Geometry: see drawing. Coordinates: mm, zero at the bounding-box minimum. A direction names the side the tool comes from. Give positions to 0.01 mm unless a question says otherwise; leave off trailing zeros. Loops run counter-clockwise (first coordinate to the right, second up) from the corner with the lowest first, then second, coordinate; pieces in that order, holes last. Notation, with made-up numbers: (65.25, 36.25) - (108.25, 36.25) arc R36 ccw to (108.25, 72.25) - close; hole circle Ø4 at (-11.75, 47.5). An arc over 180 degrees is marked (long way). One line per question, with ' | ' between items. Start each with the question number.
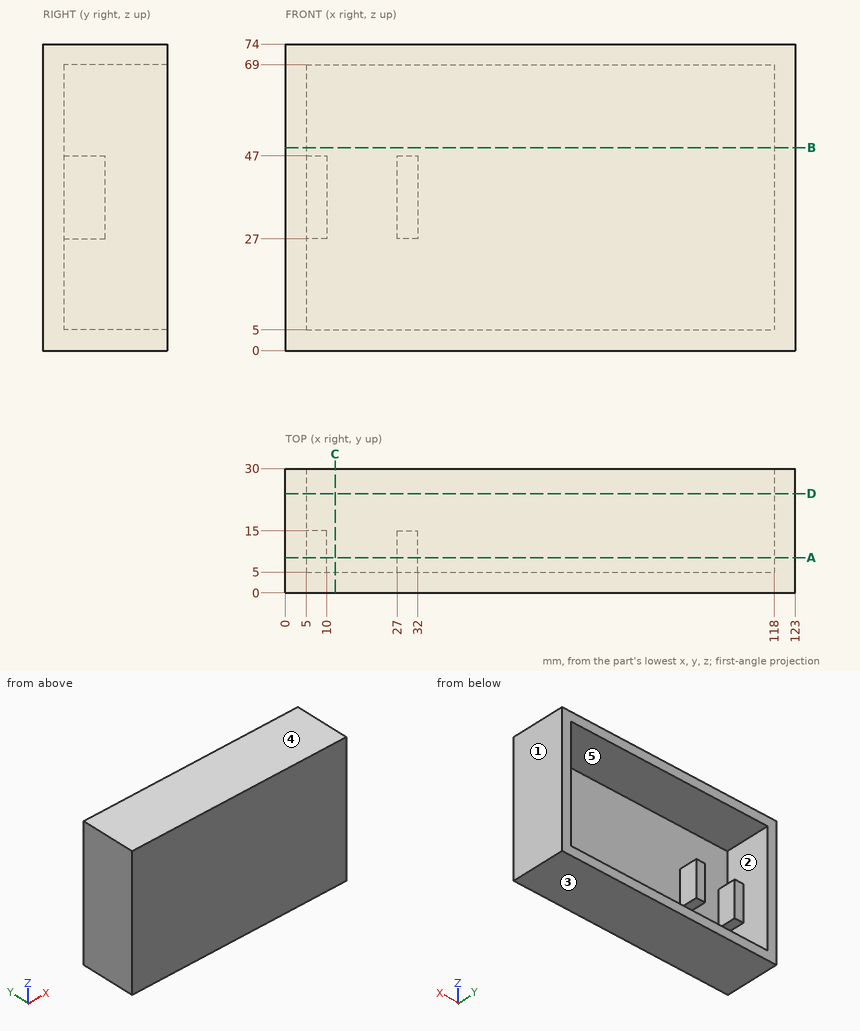
Q1. First-contact query: pin 1 (2.5 mm diameter, centred on x = 29, y = 11, fed in from -Z); pin 2 (6 mm diameter, centred on x = 68.5, z = 46.5, fed in from +Y); pin 3 (1.5 mm diameter, centred on x = 7.5, z = 37, fed in from +Y). Flat tips, straight axial feed; report the tip coordinate or a pass-through.
Q2. Section C-C, the plane x = 12. Output: boundary loops of the cut face in (y, z).
Q3. Access query for the marked faces 4 and 5. Directions: +Z, -Z, +X, -X, +Y, -Y. A direction counts if a zero-diameter tool reaches every point of the face in a straight line with its end or side. Return the directions, or none.
Q4. Draft query along Z for the marked faces 1, 2 and 3. Return one class per face: +Z half, -Z half, draft (parallel to the pull), parting line (faces both ways), or undercut.
Q5. Section B-B, the plane z = 49. Output: boundary loops of the cut face in (x, y), plus the area to 3 significant figures.
Q6. Line query: L1, parallel to X at y = 12.25, z = 45.5; L2, parallel to X at y = 8.75, z = 51; L3, parallel to Z at x = 39.5, y = 26. Output: solid intervals per line, ascending. Write a range as from..to.
Q7. Section A-A, the plane y = 8.5. Output: boundary loops of the cut face in (x, z), plus the area to 3 significant figures.
Q8. Section D-D, the plane y = 24. Output: boundary loops of the cut face in (x, z).
Solved:
1) pin 1: stops at z = 0 | pin 2: stops at y = 5 | pin 3: stops at y = 15
2) outline: (0, 0) - (30, 0) - (30, 5) - (5, 5) - (5, 69) - (30, 69) - (30, 74) - (0, 74) - close
3) face 4: +Z, +X, -X, +Y, -Y | face 5: +Y
4) face 1: draft | face 2: undercut | face 3: -Z half
5) outline: (0, 0) - (123, 0) - (123, 30) - (118, 30) - (118, 5) - (5, 5) - (5, 30) - (0, 30) - close | area: 865 mm²
6) L1: x = 0..10, 27..32, 118..123 | L2: x = 0..5, 118..123 | L3: z = 0..5, 69..74
7) outline: (0, 0) - (123, 0) - (123, 74) - (0, 74) - close; (27, 27) - (32, 27) - (32, 47) - (27, 47) - close; hole (5, 5) - (118, 5) - (118, 69) - (5, 69) - (5, 47) - (10, 47) - (10, 27) - (5, 27) - close | area: 2,070 mm²
8) outline: (0, 0) - (123, 0) - (123, 74) - (0, 74) - close; hole (5, 5) - (118, 5) - (118, 69) - (5, 69) - close
